from build123d import *

# Parameters (mm, degrees)
F1_DEPTH = 14
F2_R     = 7
F3_DEPTH = 14
F4_R     = 5


with BuildPart() as f1:
    # F0 (on Front) → F1 (new body)
    with BuildSketch(Plane.XZ):
        with BuildLine():
            Line((27, 17), (-27, 17))
            ThreePointArc((-27, 17), (-44, 0), (-27, -17))
            Line((-27, -17), (27, -17))
            Line((27, -17), (27, 17))
        make_face()
        with BuildLine():
            Line((-3, -7), (-27, -7))
            ThreePointArc((-27, -7), (-34, 0), (-27, 7))
            Line((-27, 7), (-3, 7))
            ThreePointArc((-3, 7), (4, 0), (-3, -7))
        make_face(mode=Mode.SUBTRACT)
    extrude(amount=F1_DEPTH)

    # F2 (on face) → F3 (join)
    with BuildSketch(Plane.YZ.offset(27)):
        with BuildLine():
            Line((-28, -17), (0, -17))
            Line((0, -17), (0, 17))
            Line((0, 17), (-28, 17))
            ThreePointArc((-28, 17), (-45, 0), (-28, -17))
        make_face()
        with Locations((-28, 0)):
            Circle(F2_R, mode=Mode.SUBTRACT)
    extrude(amount=-F3_DEPTH)

    # F4
    f4_edges = [f1.edges().sort_by_distance(p)[0] for p in [
        (13, -14, 0),
    ]]
    fillet(f4_edges, radius=F4_R)


solid = f1.part
The listing builds one solid part. Answer for the finished solid, in the listing's coordinates (mm). A direction names the side the tool comes from. Give positions to 0.01 mm unless a question says otherwise; leave off trailing zeros. Loops run counter-clockwise (first coordinate to the right, second up) from the corner with the lowest first, then second, coordinate; pieces in that order, holes last. Notation, with made-up numbers: (60, 15) - (119, 15) arc R33 cw to (119, 53) - close; hole circle Ø2 at (52.5, 42). An arc over 180 degrees is marked (long way). Write each question's results on one line, items separated by ' | '.
1. For a pull along X with two mould halves and no side action, classify faces 1 (the face through (-34, -7, 0)), 2 (the face through (-44, -7, 0)), 3 (the face through (20, -45, 0)) as +X half, -X half, draft (parallel to the pull), parting line (faces both ways), or undercut.
Resolved:
face 1: undercut | face 2: -X half | face 3: draft
2. Find section B-B, the plane x = -21.5. Write down the section's boundary in (y, z).
Resolved:
outline: (-14, -17) - (0, -17) - (0, -7) - (-14, -7) - close; (-14, 7) - (0, 7) - (0, 17) - (-14, 17) - close
3. Consider probe 1 along Z at (x, y) = (18.5, -28); probe 2 along X at (y, z) = (-11.5, 0); probe 3 along X at (y, z) = (-42, 6). Determine where each line is inside the solid, lowest interval first. Write a range as from..to.
Resolved:
probe 1: z = -17..-7, 7..17 | probe 2: x = -44..-34, 4..27 | probe 3: x = 13..27
4. Which of the six approach directions +Z, -Z, +X, -X, +Y, -Y give full straight-line access (tool end or side, diameter ignored) to faces 4 (the face through (13, -35, -4)), 5 (the face through (-15, -7, 7)), 6 (the face through (6, -11, -17))?
Resolved:
face 4: +Z, -Z, -X, -Y | face 5: +Y, -Y | face 6: -Z, +X, -X, +Y, -Y
5. Flat-ended cylindrical pins translate along their axes: P1, Ø3, axis at x = -18, z = 7.5, coming from the -Y side; P2, Ø3, axis at x = 14, y = -36, coming from the +Z side; P3, Ø6, axis at y = -23.5, z = 3, coming from the -X side. Find the tip coordinate at first contact, or state that the pin passes through.
Resolved:
P1: stops at y = -14 | P2: stops at z = 15.71 | P3: stops at x = 13
6. Find section D-D, the plane y = -27. Write down the section's boundary in (x, z).
Resolved:
outline: (13, -17) - (27, -17) - (27, -6.93) - (13, -6.93) - close; (13, 6.93) - (27, 6.93) - (27, 17) - (13, 17) - close
7. Find section A-A, the plane y = -4. Write down the section's boundary in (x, z).
Resolved:
outline: (-27, -17) - (27, -17) - (27, 17) - (-27, 17) arc R17 ccw to start; hole (-27, -7) - (-3, -7) arc R7 ccw to (-3, 7) - (-27, 7) arc R7 ccw to start
8. Find section C-C, the plane z = 0. Write down the section's boundary in (x, y), then the cut area to 3 significant figures.
Resolved:
outline: (-44, -14) - (-34, -14) - (-34, 0) - (-44, 0) - close; (4, -14) - (8, -14) arc R5 cw to (13, -19) - (13, -21) - (27, -21) - (27, 0) - (4, 0) - close; (13, -45) - (27, -45) - (27, -35) - (13, -35) - close | area: 705 mm^2
